The figure shows three views and two pictorial views of one solid part (mm, origin at its lowest corner). Answer the questions. A direction names the side the tool comes from. Give positions to 0.01 mm unless a question says otherwise; leave off trailing zeros. Order: outer loops, then holes, each group sorted by start corner. A loop starts at its lowest first (then second) coordinate and runs counter-clockwise, first axis right, second up. Notation, with made-up numbers: (70, 37) - (129, 37) arc R22 cw to (129, 75) - close; hole circle Ø1 at (-9.5, 0). An arc over 180 degrees is marked (long way). Write item = value, one per line.
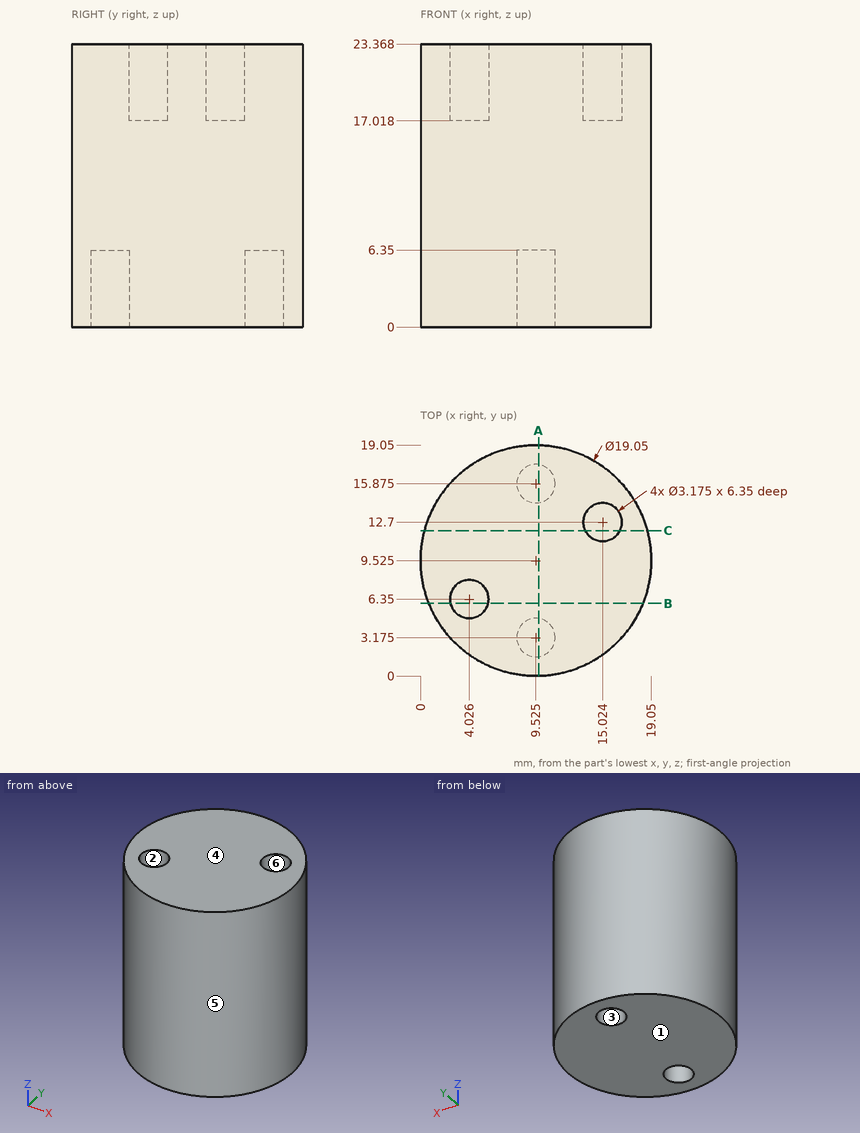
1. Determine the mould class of the marked faces 4, 5 and 6 for opening direction Y: +Y half, -Y half, draft (parallel to the pull), parting line (faces both ways), or undercut.
Recorded:
face_4 = draft
face_5 = parting line
face_6 = undercut
2. Straight lines are drawn through the part: L1, parallel to Y at x = 10.5, z = 6.25; L2, parallel to Y at x = 9.5, z = 3; L3, parallel to X at y = 12.7, z = 19.75 (1 decimal). For each, find the intervals that lie inside material, in ascending order. Write a range as [from, to].
Recorded:
L1 = [0.05, 1.92], [4.43, 14.62], [17.13, 19]
L2 = [0, 1.59], [4.76, 14.29], [17.46, 19.05]
L3 = [0.5, 13.4], [16.6, 18.5]
3. Flat-ended cylindrical pins translate along their axes: pin 1 (4 mm diameter, centred on y = 15, z = 19.5, fed in from -X); pin 2 (8 mm diameter, centred on y = 14, z = 13.5, fed in from -X); pin 3 (1.5 mm diameter, centred on x = 16.5, z = 5, fed in from +Y) (1 decimal). Find the tip coordinate at first contact, or state that the pin passes through.
Recorded:
pin_1 = 0.66
pin_2 = 0.01
pin_3 = 16.7
4. Section A-A (x = 9.75) is taken. Determine the outline of the cut face in (y, z), and give its area (3 significant figures).
Recorded:
outline = (0, 0) - (1.6, 0) - (1.6, 6.35) - (4.75, 6.35) - (4.75, 0) - (14.3, 0) - (14.3, 6.35) - (17.45, 6.35) - (17.45, 0) - (19.05, 0) - (19.05, 23.37) - (0, 23.37) - close
area = 405 mm^2
5. Section C-C (y = 12) is taken. Determine the outline of the cut face in (x, z), and give its area (3 significant figures).
Recorded:
outline = (0.33, 0) - (18.72, 0) - (18.72, 23.37) - (16.45, 23.37) - (16.45, 17.02) - (13.6, 17.02) - (13.6, 23.37) - (0.33, 23.37) - close
area = 412 mm^2
6. Section B-B (y = 6) is taken. Determine the outline of the cut face in (x, z), and give its area (3 significant figures).
Recorded:
outline = (0.68, 0) - (18.37, 0) - (18.37, 23.37) - (5.57, 23.37) - (5.57, 17.02) - (2.48, 17.02) - (2.48, 23.37) - (0.68, 23.37) - close
area = 394 mm^2
7. For the marked faces 1, 2 and 3, determine the directions among +Z, -Z, +X, -X, +Y, -Y from which every point of the face is accessible in a straight line to the end or side of a thin tool.
Recorded:
face_1 = -Z, +X, -X, +Y, -Y
face_2 = +Z
face_3 = -Z
